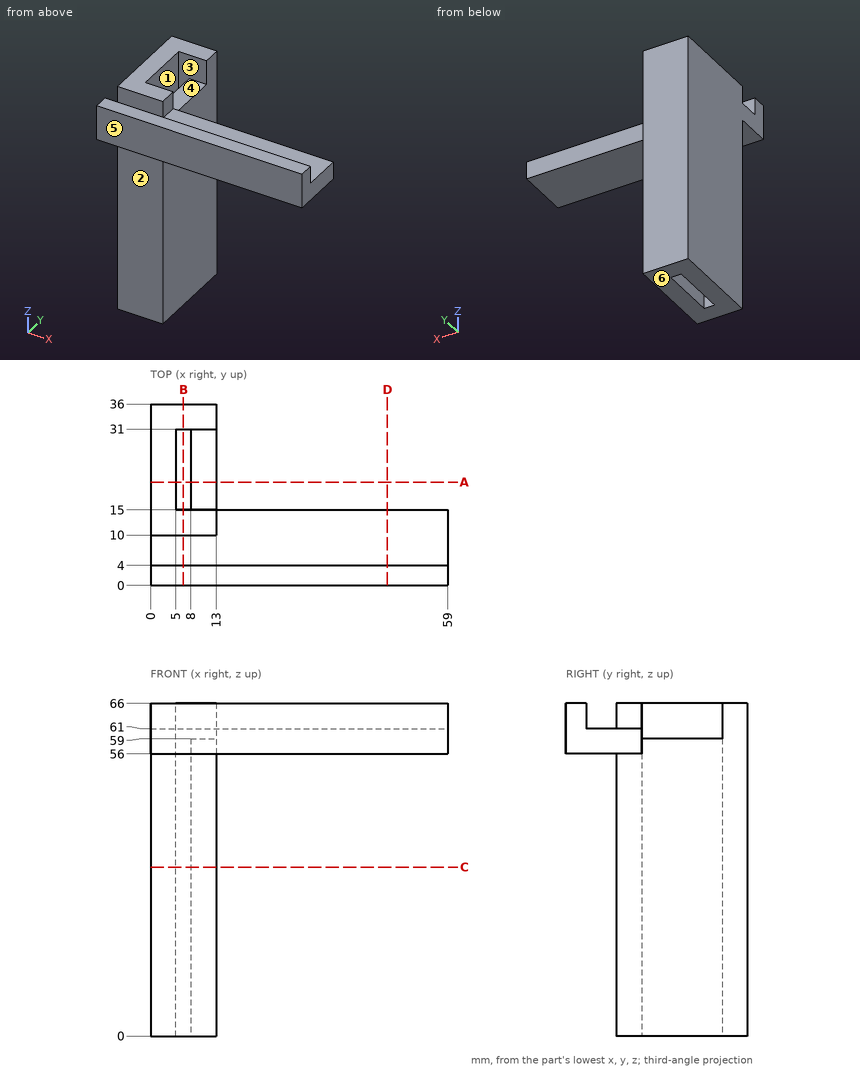
Study the drawing (mm; zero at the part's minimum x, y, z) and answer. A direction names the side the tool comes from. Coordinates: 2 decimals unless noted, no trailing zeros. Loops run counter-clockwise (first coordinate to the right, second up) from the corner with the lowest first, then second, coordinate; pieces in that order, holes last. Notation, with made-up numbers: M -34,-14.75 L -26,-14.75 A10 ccw -26,-7.75 Z; hole C 73,76 d5. An arc over 180 degrees is marked long. Answer as a JSON object with one key per item and string values. Group by question number.
Item 1: Section A-A (y = 20.5) is taken. Write down the section's boundary in (x, z), and give its area (3 significant figures).
Item 2: Section C-C (z = 33.5) is taken. Write down the section's boundary in (x, y), and give its area (3 significant figures).
Item 3: Section D-D (x = 47) is taken. Write down the section's boundary in (y, z), and give its area (3 significant figures).
Item 4: Section B-B (x = 6.5) is taken. Write down the section's boundary in (y, z), and give its area (3 significant figures).
Item 5: Consider L1, parallel to X at y = 30.5, z = 12.5; L2, parallel to Y at x = 6.5, z = 5.5; L3, parallel to Y at x = 30.5, z = 58. Determine where each line is inside the solid, lowest interval first.
Item 6: Each of these flat-tipped pins is pushed along its axis until it touches: P1, Ø1, axis at y = 10.5, z = 19.5, coming from the +X side; P2, Ø10.5, axis at x = 3.5, z = 19, coming from the -Y side; P3, Ø4, axis at x = 42.5, y = 18.5, coming from the +Z side; P4, Ø1.5, axis at x = 10.5, y = 22, coming from the +Z side. Where does it stop, or does it pass through?
Item 7: Which of the six approach directions +Z, -Z, +X, -X, +Y, -Y give full straight-line access (tool end or side, diameter ignored) to the marked faces 1, 2 and 3?
Item 8: Determine the mould class of the marked faces 4, 5 and 6 for opening direction Z: +Z half, -Z half, draft (parallel to the pull), parting line (faces both ways), or undercut.
Solved:
{
 "1": {"outline": "M 0,0 L 5,0 L 5,66 L 0,66 Z; M 8,0 L 13,0 L 13,59 L 8,59 Z", "area": "625 mm2"},
 "2": {"outline": "M 0,10 L 13,10 L 13,36 L 0,36 Z; hole M 5,15 L 8,15 L 8,31 L 5,31 Z", "area": "290 mm2"},
 "3": {"outline": "M 0,56 L 15,56 L 15,61 L 4,61 L 4,66 L 0,66 Z", "area": "95.0 mm2"},
 "4": {"outline": "M 0,56 L 10,56 L 10,0 L 15,0 L 15,66 L 10,66 L 10,61 L 4,61 L 4,66 L 0,66 Z; M 31,0 L 36,0 L 36,66 L 31,66 Z", "area": "730 mm2"},
 "5": {"L1": "x = 0 to 5, 8 to 13", "L2": "y = 10 to 15, 31 to 36", "L3": "y = 0 to 15"},
 "6": {"P1": "stops at x = 13", "P2": "stops at y = 10", "P3": "passes through", "P4": "stops at z = 59"},
 "7": {"face 1": "+Z, -Z", "face 2": "-Z, +X, -X, -Y", "face 3": "+Z"},
 "8": {"face 4": "+Z half", "face 5": "draft", "face 6": "-Z half"}
}
